from build123d import *

# Parameters (mm, degrees)
SKETCH1_R            = 15
BOSS_EXTRUDE1_DEPTH  = 27
SKETCH2_R            = 14
BOSS_EXTRUDE2_DEPTH  = 5
SKETCH3_R            = 5
BOSS_EXTRUDE3_DEPTH  = 3
SKETCH4_R            = 1.25
BOSS_EXTRUDE4_DEPTH  = 7
BOSS_EXTRUDE5_START  = 6
SKETCH5_R            = 14
BOSS_EXTRUDE5_DEPTH  = 6
BOSS_EXTRUDE6_START  = 3
SKETCH6_R            = 5
BOSS_EXTRUDE6_DEPTH  = 3
SKETCH7_W            = 26.5
SKETCH7_H            = 28
BOSS_EXTRUDE7_DEPTH  = 2.5
BOSS_EXTRUDE8_START  = 4
SKETCH8_R            = 1.25
BOSS_EXTRUDE8_DEPTH  = 4
BOSS_EXTRUDE9_START  = 1
SKETCH9_R            = 5
BOSS_EXTRUDE9_DEPTH  = 1
SKETCH10_R           = 11
BOSS_EXTRUDE10_DEPTH = 0.5
BOSS_EXTRUDE11_START = 1
SKETCH11_R           = 5
BOSS_EXTRUDE11_DEPTH = 1
BOSS_EXTRUDE12_START = 3
SKETCH12_R           = 1.25
BOSS_EXTRUDE12_DEPTH = 3
SKETCH13_R           = 1.5
CUT_EXTRUDE1_DEPTH   = 20


with BuildPart() as part:
    # Sketch1 → Boss-Extrude1 (new body)
    with BuildSketch(Plane(origin=(0, 0, 0), x_dir=(1, 0, 0), z_dir=(0, 1, 0))):
        with Locations(Location((0, 0, 0), (0, 0, 270))):
            Circle(SKETCH1_R)
    extrude(amount=BOSS_EXTRUDE1_DEPTH)

    # Sketch2 → Boss-Extrude2 (add)
    with BuildSketch(Plane(origin=(0, 27, 0), x_dir=(1, 0, 0), z_dir=(0, 1, 0))):
        with Locations(Location((0, 0, 0), (0, 0, 270))):
            Circle(SKETCH2_R)
    extrude(amount=BOSS_EXTRUDE2_DEPTH)

    # Sketch3 → Boss-Extrude3 (add)
    with BuildSketch(Plane(origin=(0, 32, 0), x_dir=(1, 0, 0), z_dir=(0, 1, 0))):
        with Locations(Location((0, 0, 0), (0, 0, 270))):
            Circle(SKETCH3_R)
    extrude(amount=BOSS_EXTRUDE3_DEPTH)

    # Sketch4 → Boss-Extrude4 (add)
    with BuildSketch(Plane(origin=(0, 35, 0), x_dir=(1, 0, 0), z_dir=(0, 1, 0))):
        with Locations(Location((0, 0, 0), (0, 0, 270))):
            Circle(SKETCH4_R)
    extrude(amount=BOSS_EXTRUDE4_DEPTH)

    # Sketch5 → Boss-Extrude5 (add)
    with BuildSketch(Plane.XZ.offset(BOSS_EXTRUDE5_START)):
        with Locations(Location((0, 0, 0), (0, 0, 90))):
            Circle(SKETCH5_R)
    extrude(amount=-BOSS_EXTRUDE5_DEPTH)

    # Sketch6 → Boss-Extrude6 (add)
    with BuildSketch(Plane.XZ.offset(6).offset(BOSS_EXTRUDE6_START)):
        with Locations(Location((0, 0, 0), (0, 0, 90))):
            Circle(SKETCH6_R)
    extrude(amount=-BOSS_EXTRUDE6_DEPTH)

    # Sketch7 → Boss-Extrude7 (add)
    with BuildSketch(Plane.XZ.offset(6)):
        with Locations((-13.25, 0)):
            Rectangle(SKETCH7_W, SKETCH7_H)
    extrude(amount=BOSS_EXTRUDE7_DEPTH)

    # Sketch8 → Boss-Extrude8 (add)
    with BuildSketch(Plane.XZ.offset(9).offset(BOSS_EXTRUDE8_START)):
        with Locations(Location((0, 0, 0), (0, 0, 90))):
            Circle(SKETCH8_R)
    extrude(amount=-BOSS_EXTRUDE8_DEPTH)

    # Sketch9 → Boss-Extrude9 (add)
    with BuildSketch(Plane.XZ.offset(13).offset(BOSS_EXTRUDE9_START)):
        with Locations(Location((0, 0, 0), (0, 0, 270))):
            Circle(SKETCH9_R)
    extrude(amount=-BOSS_EXTRUDE9_DEPTH)

    # Sketch10 → Boss-Extrude10 (add)
    with BuildSketch(Plane.XZ.offset(14)):
        with Locations(Location((0, 0, 0), (0, 0, 270))):
            Circle(SKETCH10_R)
    extrude(amount=BOSS_EXTRUDE10_DEPTH)

    # Sketch11 → Boss-Extrude11 (add)
    with BuildSketch(Plane.XZ.offset(14.5).offset(BOSS_EXTRUDE11_START)):
        with Locations(Location((0, 0, 0), (0, 0, 270))):
            Circle(SKETCH11_R)
    extrude(amount=-BOSS_EXTRUDE11_DEPTH)

    # Sketch12 → Boss-Extrude12 (add)
    with BuildSketch(Plane.XZ.offset(15.5).offset(BOSS_EXTRUDE12_START)):
        with Locations(Location((0, 0, 0), (0, 0, 90))):
            Circle(SKETCH12_R)
    extrude(amount=-BOSS_EXTRUDE12_DEPTH)

    # Sketch13 → Cut-Extrude1 (cut)
    with BuildSketch(Plane(origin=(0, 32, 0), x_dir=(1, 0, 0), z_dir=(0, 1, 0))):
        with Locations(Location((0, 8, 0), (0, 0, 270))):
            Circle(SKETCH13_R)
        with Locations(Location((0, -8, 0), (0, 0, 270))):
            Circle(SKETCH13_R)
    extrude(amount=-CUT_EXTRUDE1_DEPTH, mode=Mode.SUBTRACT)


solid = part.part
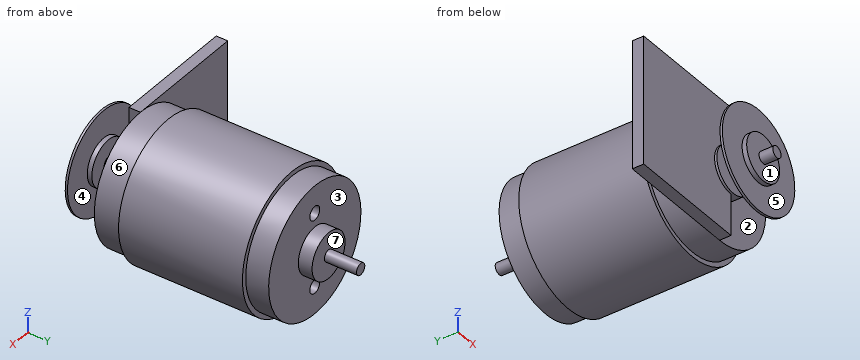
Can you work these out from the model? Positions are in its coordinate system, mm. Face numbers are marked on the shaded views. A direction names the side the tool comes from. Round coordinates to 2 decimals unless told otherwise and drop trailing zeros. Write each loop counter-clockwise with the first axis right and the second up, starting at its lowest first coordinate (ties: lowest second). Pieces come first, ordered by that corner, then holes. Notation, with made-up numbers: (63, 10.25) -> (92, 10.25) arc R16 cw to (92, 20.25) -> close; hole circle Ø5 at (55, 73.5). An arc over 180 degrees is marked (long way). Use one line per item in the form item = value. Start each with the question number.
Q1. Imagine slicing it at B-B (x = 8). Please give me the cut outline in (y, z), then the cut area to 3 significant figures.
Q2. I'm going to push flat-ended pins straight in: P1, Ø1, axis at x = -9.5, y = 17, coming from the -Z side; P2, Ø5, axis at x = -9.5, y = 25, coming from the +Z side; P3, Ø2, axis at y = -7.5, z = -8, coming from the +X side. Where does each tip first touch, or does it pass through?
Q3. Which directions (+Z, -Z, +X, -X, +Y, -Y) give clear straight access to the entire face, cutting with the end or side of a thin tool? Please do the marked faces 1, 2, 3 and 4.
Q4. We'd pull the mould along Y, two halves only. Please class the marked faces 5, 6 and 7: +Y half, -Y half, draft (parallel to the pull), parting line (faces both ways), or undercut.
Q5. Imagine slicing it at A-A (z = -8). Please give me the cut outline in (x, y), then the cut area to 3 significant figures.
Q6. If I drill on probe 1 along Y at (x, z) = (-4, 3.5); probe 2 along Y at (x, z) = (-14, 1); probe 3 along X at (y, z) = (10.5, 0.25), over which ranges is the centre line in solid material (lowest first)? Write a range as [from, to].
Q7. Imagine slicing it at D-D (z = 12.5). Please give me the cut outline in (x, y).
Q8. Imagine slicing it at C-C (y = 21). Please give me the cut outline in (x, z).
Worked out:
q1.outline = (-14.5, -7.55) -> (-14, -7.55) -> (-14, 7.55) -> (-14.5, 7.55) -> close; (-6, -11.49) -> (0, -11.49) -> (0, -12.69) -> (27, -12.69) -> (27, -11.49) -> (32, -11.49) -> (32, 11.49) -> (27, 11.49) -> (27, 12.69) -> (0, 12.69) -> (0, 11.49) -> (-6, 11.49) -> close
q1.area = 945 mm^2
q2.P1 = -12
q2.P2 = 13.27
q2.P3 = 0
q3.face_1 = -Y
q3.face_2 = +X
q3.face_3 = +Y
q3.face_4 = none
q4.face_5 = -Y half
q4.face_6 = undercut
q4.face_7 = +Y half
q5.outline = (-26.5, -8.5) -> (0, -8.5) -> (0, -6) -> (11.49, -6) -> (11.49, 0) -> (12.69, 0) -> (12.69, 27) -> (11.49, 27) -> (11.49, 32) -> (1.5, 32) -> (1.5, 12) -> (-1.5, 12) -> (-1.5, 32) -> (-11.49, 32) -> (-11.49, 27) -> (-12.69, 27) -> (-12.69, 0) -> (-11.49, 0) -> (-11.49, -6) -> (-26.5, -6) -> close; (-7.55, -14.5) -> (7.55, -14.5) -> (7.55, -14) -> (-7.55, -14) -> close
q5.area = 952 mm^2
q6.probe_1 = [-14.5, -14], [-8.5, 32]
q6.probe_2 = [-8.5, -6], [0, 27]
q6.probe_3 = [-15, 15]
q7.outline = (-26.5, -8.5) -> (0, -8.5) -> (0, -6) -> (6.3, -6) -> (6.3, 0) -> (8.29, 0) -> (8.29, 27) -> (6.3, 27) -> (6.3, 32) -> (-6.3, 32) -> (-6.3, 27) -> (-8.29, 27) -> (-8.29, 0) -> (-6.3, 0) -> (-6.3, -6) -> (-26.5, -6) -> close
q8.outline = circle Ø30 at (0, 0); hole circle Ø3 at (0, -8); hole circle Ø3 at (0, 8)
